from build123d import *

# Parameters (mm, degrees)
SKETCH1_R           = 1.6
SKETCH1_R_2         = 1.5875
BOSS_EXTRUDE1_DEPTH = 2.54
SKETCH2_W           = 82.55
SKETCH2_H           = 17.78
BOSS_EXTRUDE2_DEPTH = 2.54


with BuildPart() as part:
    # Sketch1 → Boss-Extrude1 (new body)
    with BuildSketch(Plane(origin=(0, 10.380200841, 0), x_dir=(1, 0, 0), z_dir=(0, 1, 0))):
        with BuildLine():
            Line((-38.220672856, -111.749766717), (-120.770672856, -111.749766717))
            Line((-120.770672856, -111.749766717), (-172.786827669, -75.327663008))
            Line((-172.786827669, -75.327663008), (-172.786827669, -66.437663008))
            Line((-172.786827669, -66.437663008), (-139.027490416, -66.437663008))
            ThreePointArc((-139.027490416, -66.437663008), (-79.495672856, -100.970943664), (-19.963855297, -66.437663008))
            Line((-19.963855297, -66.437663008), (13.795481956, -66.437663008))
            Line((13.795481956, -66.437663008), (13.795481956, -75.327663008))
            Line((13.795481956, -75.327663008), (-38.220672856, -111.749766717))
        make_face()
        with Locations((-17.327095379, -72.094107722)):
            Circle(SKETCH1_R, mode=Mode.SUBTRACT)
        with Locations((-141.664250334, -72.094107722)):
            Circle(SKETCH1_R, mode=Mode.SUBTRACT)
        with Locations((-94.127447008, -103.699839694)):
            Circle(SKETCH1_R, mode=Mode.SUBTRACT)
        with Locations((-64.863898705, -103.699839694)):
            Circle(SKETCH1_R, mode=Mode.SUBTRACT)
        with Locations((-120.770672856, -106.669766717)):
            Circle(SKETCH1_R_2, mode=Mode.SUBTRACT)
        with Locations((-167.256455611, -74.120071212)):
            Circle(SKETCH1_R_2, mode=Mode.SUBTRACT)
        with Locations((8.265109898, -74.120071212)):
            Circle(SKETCH1_R_2, mode=Mode.SUBTRACT)
        with Locations((-38.220672856, -106.669766717)):
            Circle(SKETCH1_R_2, mode=Mode.SUBTRACT)
    extrude(amount=BOSS_EXTRUDE1_DEPTH)

    # Sketch2 → Boss-Extrude2 (add)
    with BuildSketch(Plane.XY.offset(111.749766717)):
        with Locations((-79.495672856, 4.030200841)):
            Rectangle(SKETCH2_W, SKETCH2_H)
    extrude(amount=BOSS_EXTRUDE2_DEPTH)


solid = part.part
Here's how the part is built. I have some questions about the finished solid (model axes, mm). A direction names the side the tool comes from. Coordinates: 2 decimals unless noted, no trailing zeros. Order: outer loops, then holes, each group sorted by start corner. A loop starts at its lowest first (then second) coordinate and runs counter-clockwise, first axis right, second up.
Item 1: If we section it at B-B on y = -1.75: List the corners of the cut face in (x, z) for me.
Result sheet:
outline: (-120.77, 111.75) - (-38.22, 111.75) - (-38.22, 114.29) - (-120.77, 114.29) - close
Item 2: For faces 5 (the face through (-64.004, 11.632, 102.351)), 6 (the face through (-80, 3, 111.75)), which set-ups out of +Z, -Z, +X, -X, +Y, -Y let a thin tool reach every point of the face, with its end or its side?
Result sheet:
face 5: +Y, -Y
face 6: -Z, +X, -X, -Y
Item 3: If we mould it in two halves opening along X, with no side actions, what happens to faces 1 (the face through (7.92, 11.63, 75.67)), 2 (the face through (-80.505, 11.632, 100.964)), 3 (the face through (-81, 12.92, 106)), 4 (the face through (-11.848, 11.632, 93.284))? For each: +X half, -X half, draft (parallel to the pull), parting line (faces both ways), or undercut.
Result sheet:
face 1: undercut
face 2: undercut
face 3: draft
face 4: +X half
Item 4: For P1, Ø4, axis at x = -167.26, z = 74.12, coming from the -Y side; P2, Ø1.3, axis at y = 8, z = 112.5, coming from the -X side; P3, Ø3, axis at y = 3, z = 113, coming from the +X side, each with a flat end and sliding along its axis, tell me the tip position at first contact or that it passes through.
Result sheet:
P1: stops at y = 10.38
P2: stops at x = -120.77
P3: stops at x = -38.22
Item 5: I need wall thicknesses on line 1 (Y direction, x = -92.5, z = 111); line 2 (X direction, y = 11.5, z = 104); line 3 (Z direction, x = -40, y = 4). Which ranges of each line are inside material? Lowest first, please.
Result sheet:
line 1: y = 10.38 to 12.92
line 2: x = -131.84 to -95.7, -92.56 to -66.44, -63.29 to -27.15
line 3: z = 111.75 to 114.29
Item 6: If we section it at D-D on z = 92: List the corners of the cut face in (x, y) for me, plus the area to 3 significant figures.
Result sheet:
outline: (-148.98, 10.38) - (-113.41, 10.38) - (-113.41, 12.92) - (-148.98, 12.92) - close; (-45.58, 10.38) - (-10.02, 10.38) - (-10.02, 12.92) - (-45.58, 12.92) - close
area: 181 mm2
Item 7: If we section it at C-C on x = -83: List the corners of the cut face in (y, z) for me, plus the area to 3 significant figures.
Result sheet:
outline: (-4.86, 111.75) - (10.38, 111.75) - (10.38, 100.88) - (12.92, 100.88) - (12.92, 114.29) - (-4.86, 114.29) - close
area: 72.8 mm2
Item 8: If we section it at A-A on z = 80: List the corners of the cut face in (x, y) for me.
Result sheet:
outline: (-166.11, 10.38) - (-128.86, 10.38) - (-128.86, 12.92) - (-166.11, 12.92) - close; (-30.13, 10.38) - (7.12, 10.38) - (7.12, 12.92) - (-30.13, 12.92) - close
